Can you work these out from the model? Positions are in its coordinate system, mm. A direction names the side the tool comes from. Coordinates: 2 decimals unless noted, no trailing zeros. Write each loop counter-clockwise with the first axis right and the second up, starting at its lowest first coordinate (ties: lowest second). Pieces come first, ordered by that corner, then holes. Notation, with made-up numbers: M 64.25,-11.75 L 101.25,-11.75 A13 cw 101.25,3.25 Z; hole C 71.25,67 d8. An arc over 180 degrees is marked long. Answer as a JSON object with one key per item and string values. Group by question number.
from build123d import *

# Parameters (mm, degrees)
SKETCH_1_W          = 32.5
SKETCH_1_H          = 25.5
EXTRUDE_1_DEPTH     = 3
EXTRUDE_2_DEPTH     = 1.5
SKETCH_5_R          = 1.4
EXTRUDE_3_DEPTH     = 3.7
SKETCH_6_R          = 0.725
EXTRUDE_4_DEPTH     = 1
SKETCH_7_R          = 1
CUT_EXTRUDE_1_DEPTH = 10
SKETCH_8_R          = 2
CUT_EXTRUDE_2_DEPTH = 1
FILLET_1_R          = 2
SKETCH_9_R          = 2.65
EXTRUDE_5_DEPTH     = 2
SKETCH_11_R         = 1.05
CUT_EXTRUDE_4_DEPTH = 100
SKETCH_12_R         = 1.425
CUT_EXTRUDE_5_DEPTH = 4
FILLET_2_R          = 0.3
CUT_EXTRUDE_8_DEPTH = 2
CUT_EXTRUDE_9_DEPTH = 1.5
EXTRUDE_6_DEPTH     = 6.4
FILLET_3_R          = 2
FILLET_5_R          = 1
FILLET_6_R          = 0.4


with BuildPart() as part:
    # 草图1 → 凸台-拉伸1 (new body)
    with BuildSketch(Plane(origin=(0, 0, 0), x_dir=(1, 0, 0), z_dir=(0, 1, 0))):
        Rectangle(SKETCH_1_W, SKETCH_1_H)
    extrude(amount=EXTRUDE_1_DEPTH)

    # 草图2 → 凸台-拉伸2 (add)
    with BuildSketch(Plane(origin=(0, 3, 0), x_dir=(1, 0, 0), z_dir=(0, 1, 0))):
        Polygon((-5.4, 5.35), (5.4, 5.35), (5.4, -7.55), (4.4, -7.55), (4.4, 4.35), (-4.4, 4.35), (-4.4, -7.55), (-5.4, -7.55), align=None)
    extrude(amount=EXTRUDE_2_DEPTH)

    # 草图5 → 凸台-拉伸3 (add)
    with BuildSketch(Plane(origin=(0, 3, 0), x_dir=(1, 0, 0), z_dir=(0, 1, 0))):
        with Locations(Location((12.5, 5.5, 0), (0, 0, 270))):
            Circle(SKETCH_5_R)
        with Locations(Location((12.5, -5.5, 0), (0, 0, 90))):
            Circle(SKETCH_5_R)
        with Locations(Location((-12.5, -5.5, 0), (0, 0, 270))):
            Circle(SKETCH_5_R)
        with Locations(Location((-12.5, 5.5, 0), (0, 0, 90))):
            Circle(SKETCH_5_R)
    extrude(amount=EXTRUDE_3_DEPTH)

    # 草图6 → 凸台-拉伸4 (add)
    with BuildSketch(Plane(origin=(0, 6.7, 0), x_dir=(1, 0, 0), z_dir=(0, 1, 0))):
        with Locations(Location((-12.5, -5.5, 0), (0, 0, 270))):
            Circle(SKETCH_6_R)
        with Locations(Location((-12.5, 5.5, 0), (0, 0, 270))):
            Circle(SKETCH_6_R)
        with Locations(Location((12.5, 5.5, 0), (0, 0, 270))):
            Circle(SKETCH_6_R)
        with Locations(Location((12.5, -5.5, 0), (0, 0, 270))):
            Circle(SKETCH_6_R)
    extrude(amount=EXTRUDE_4_DEPTH)

    # 草图7 → 切除-拉伸1 (cut)
    with BuildSketch(Plane(origin=(0, 3, 0), x_dir=(1, 0, 0), z_dir=(0, 1, 0))):
        with Locations(Location((13.5, 10, 0), (0, 0, 270))):
            Circle(SKETCH_7_R)
        with Locations(Location((-13.5, 10, 0), (0, 0, 270))):
            Circle(SKETCH_7_R)
        with Locations(Location((-13.5, -10, 0), (0, 0, 270))):
            Circle(SKETCH_7_R)
        with Locations(Location((13.5, -10, 0), (0, 0, 270))):
            Circle(SKETCH_7_R)
    extrude(amount=-CUT_EXTRUDE_1_DEPTH, mode=Mode.SUBTRACT)

    # 草图8 → 切除-拉伸2 (cut)
    with BuildSketch(Plane.XZ):
        with Locations(Location((-13.5, 10, 0), (0, 0, 270))):
            Circle(SKETCH_8_R)
        with Locations(Location((13.5, 10, 0), (0, 0, 270))):
            Circle(SKETCH_8_R)
        with Locations(Location((13.5, -10, 0), (0, 0, 270))):
            Circle(SKETCH_8_R)
        with Locations(Location((-13.5, -10, 0), (0, 0, 270))):
            Circle(SKETCH_8_R)
    extrude(amount=-CUT_EXTRUDE_2_DEPTH, mode=Mode.SUBTRACT)

    # 圆角1
    fillet_1_edges = [part.edges().sort_by_distance(p)[0] for p in [
        (16.25, 1.5, 12.75),
        (-16.25, 1.5, 12.75),
        (-16.25, 1.5, -12.75),
        (16.25, 1.5, -12.75),
    ]]
    fillet(fillet_1_edges, radius=FILLET_1_R)

    # 草图9 → 凸台-拉伸5 (add)
    with BuildSketch(Plane(origin=(0, 3, 0), x_dir=(1, 0, 0), z_dir=(0, 1, 0))):
        with Locations(Location((8.5, 7.75, 0), (0, 0, 270))):
            Circle(SKETCH_9_R)
        with Locations(Location((-8.5, 7.75, 0), (0, 0, 90))):
            Circle(SKETCH_9_R)
        with Locations(Location((-8.5, -7.75, 0), (0, 0, 270))):
            Circle(SKETCH_9_R)
        with Locations(Location((8.5, -7.75, 0), (0, 0, 90))):
            Circle(SKETCH_9_R)
    extrude(amount=EXTRUDE_5_DEPTH)

    # 草图11 → 切除-拉伸4 (cut)
    with BuildSketch(Plane(origin=(0, 5, 0), x_dir=(1, 0, 0), z_dir=(0, 1, 0))):
        with Locations(Location((-8.5, 7.75, 0), (0, 0, 270))):
            Circle(SKETCH_11_R)
        with Locations(Location((-8.5, -7.75, 0), (0, 0, 270))):
            Circle(SKETCH_11_R)
        with Locations(Location((8.5, -7.75, 0), (0, 0, 270))):
            Circle(SKETCH_11_R)
        with Locations(Location((8.5, 7.75, 0), (0, 0, 270))):
            Circle(SKETCH_11_R)
    extrude(amount=-CUT_EXTRUDE_4_DEPTH, mode=Mode.SUBTRACT)

    # 草图12 → 切除-拉伸5 (cut)
    with BuildSketch(Plane(origin=(0, 5, 0), x_dir=(1, 0, 0), z_dir=(0, 1, 0))):
        with Locations(Location((-8.5, 7.75, 0), (0, 0, 270))):
            Circle(SKETCH_12_R)
        with Locations(Location((8.5, 7.75, 0), (0, 0, 270))):
            Circle(SKETCH_12_R)
        with Locations(Location((-8.5, -7.75, 0), (0, 0, 270))):
            Circle(SKETCH_12_R)
        with Locations(Location((8.5, -7.75, 0), (0, 0, 270))):
            Circle(SKETCH_12_R)
    extrude(amount=-CUT_EXTRUDE_5_DEPTH, mode=Mode.SUBTRACT)

    # 圆角2
    fillet_2_edges = [part.edges().sort_by_distance(p)[0] for p in [
        (-12.5, 7.7, 4.775),
        (-12.5, 7.7, -6.225),
        (12.5, 7.7, -6.225),
        (12.5, 7.7, 4.775),
    ]]
    fillet(fillet_2_edges, radius=FILLET_2_R)

    # 草图15 → 切除-拉伸8 (cut)
    with BuildSketch(Plane(origin=(0, 3, 0), x_dir=(1, 0, 0), z_dir=(0, 1, 0))):
        Polygon((-4.4, 4.35), (4.4, 4.35), (4.4, -7.55), (3.2, -7.55), (3.2, -12.75), (-3.2, -12.75), (-3.2, -7.55), (-4.4, -7.55), align=None)
    extrude(amount=-CUT_EXTRUDE_8_DEPTH, mode=Mode.SUBTRACT)

    # 草图17 → 切除-拉伸9 (cut)
    with BuildSketch(Plane(origin=(0, 4.5, 0), x_dir=(1, 0, 0), z_dir=(0, 1, 0))):
        Polygon((-4.4, -7.55), (-4.4, 4.35), (4.4, 4.35), (4.4, -7.55), (5.4, -7.55), (5.4, 5.35), (-5.4, 5.35), (-5.4, -7.55), align=None)
    extrude(amount=-CUT_EXTRUDE_9_DEPTH, mode=Mode.SUBTRACT)

    # 草图18 → 凸台-拉伸6 (add)
    with BuildSketch(Plane.ZY.offset(-3.2)):
        Polygon((12.75, 1), (9.75, 1), (12.25, 2.6), (12.75, 2.6), align=None)
    extrude(amount=EXTRUDE_6_DEPTH)

    # 圆角3
    fillet_3_edges = [part.edges().sort_by_distance(p)[0] for p in [
        (0, 1, 9.75),
    ]]
    fillet(fillet_3_edges, radius=FILLET_3_R)

    # 圆角5
    fillet_5_edges = [part.edges().sort_by_distance(p)[0] for p in [
        (0, 2.6, 12.25),
    ]]
    fillet(fillet_5_edges, radius=FILLET_5_R)

    # 圆角6
    fillet_6_edges = [part.edges().sort_by_distance(p)[0] for p in [
        (3.2, 2, 7.55),
        (-3.2, 2, 7.55),
    ]]
    fillet(fillet_6_edges, radius=FILLET_6_R)


solid = part.part
Q1. If we section it at A-A on x = 8.5: List the corners of the cut face in (y, z) for me (3 decimals).
Q2. We'd pull the mould along X, two halves only. Please class faces 4 (the cylindrical face through (15.65, 1.52, 12.18)), 5 (the cylindrical face through (12.059, 7.045, -6.075)), 6 (the flat face through (-12.5, 7.7, -5.5)): pulls with the +X half, pulls with the -X half, needs draft (parallel to the pull), parting line crosses it, or undercut.
Q3. If we section it at B-B on z = 0.75: List the corners of the cut face in (x, y) for me.
Q4. On a 3-axis mill with a long thin cutter (end or side, diameter ignored), from which of +Z, -Z, +X, -X, +Y, -Y can I reach the whole of each face in a straight line? I mean faces 1 (the flat face through (12.5, 6.7, 4.6)), 2 (the cylindrical face through (15.483, 0.493, 10.26)), 3 (the flat face through (16.25, 1, 0)). Say none if no direction works.
Q5. Please list where these lines run through material, in increasing order: L1, parallel to X at y = 0.2, z = 7.75; L2, parallel to X at y = 1.7, z = 10; L3, parallel to X at y = 2.4, z = -7.75 (3 decimals).
Q6. If we section it at C-C on y = 6: List the corners of the cut face in (x, z) for me.
Q7. If we section it at D-D on x = 2: List the corners of the cut face in (y, z) for me.
Q8. Will these pins go through, and if not, where does the flat tip stop? pin 1 (3 mm diameter, centred on x = -6, z = 6.5, fed in from +Y); pin 2 (1.2 mm diameter, centred on x = -13, z = -10, fed in from -Y); pin 3 (2.5 mm diameter, centred on x = -8.5, z = -7.75, fed in from +Y).
Reply:
{
 "1": {"outline": "M 0,-12.75 L 3,-12.75 L 3,-10.4 L 5,-10.4 L 5,-9.175 L 1,-9.175 L 1,-8.8 L 0,-8.8 Z; M 0,-6.7 L 1,-6.7 L 1,-6.325 L 5,-6.325 L 5,-5.1 L 3,-5.1 L 3,5.1 L 5,5.1 L 5,6.325 L 1,6.325 L 1,6.7 L 0,6.7 Z; M 0,8.8 L 1,8.8 L 1,9.175 L 5,9.175 L 5,10.4 L 3,10.4 L 3,12.75 L 0,12.75 Z"},
 "2": {"face 4": "pulls with the +X half", "face 5": "undercut", "face 6": "needs draft"},
 "3": {"outline": "M -16.25,0 L 16.25,0 L 16.25,3 L 4.4,3 L 4.4,1 L -4.4,1 L -4.4,3 L -16.25,3 Z"},
 "4": {"face 1": "+Y", "face 2": "-Y", "face 3": "+Z, -Z, +X, +Y, -Y"},
 "5": {"L1": "-16.25 to -9.55, -7.45 to 7.45, 9.55 to 16.25", "L2": "-16.25 to -14.5, -12.5 to -3.2, 3.2 to 12.5, 14.5 to 16.25", "L3": "-16.25 to -9.925, -7.075 to 7.075, 9.925 to 16.25"},
 "6": {"outline": "C -12.5,-5.5 d2.8; C -12.5,5.5 d2.8; C 12.5,-5.5 d2.8; C 12.5,5.5 d2.8"},
 "7": {"outline": "M 0,-12.75 L 3,-12.75 L 3,-4.35 L 1,-4.35 L 1,9.16 A2 cw 1.32,10.24 L 2.44,12 A1 ccw 2.6,12.54 L 2.6,12.75 L 0,12.75 Z"},
 "8": {"pin 1": "y = 5", "pin 2": "y = 1", "pin 3": "y = 1"}
}
